Geometry: final body of the model. Coordinates: model frame, mm. Round coordinates to 2 decimals unless told otherwise and drop trailing zeros. Loops run counter-clockwise (first coordinate to the right, second up) from the corner with the lowest first, then second, coordinate; pieces in that order, holes last. Notation, with made-up numbers: (89, 26.5) -> (96, 26.5) arc R12 ccw to (96, 30.5) -> close; hole circle Ø3 at (83.25, 12.25). An arc over 180 degrees is marked (long way). Answer in a Markdown table with one row per item.
```python
from build123d import *

# Parameters (mm, degrees)
F0_W     = 146.750048
F0_H     = 97.573176
F1_DEPTH = 63.5
F3_DEPTH = 97.574176
F5_DEPTH = 97.574176


with BuildPart() as f1:
    # F0 (on Top) → F1 (new body)
    with BuildSketch(Plane.XY):
        Rectangle(F0_W, F0_H)
    extrude(amount=F1_DEPTH)

    # F2 (on face) → F3 (cut, through all)
    with BuildSketch(Plane.XZ.offset(48.786588)):
        Polygon((73.375024, 63.5), (0, 63.5), (73.375024, 0), align=None)
    extrude(amount=-F3_DEPTH, mode=Mode.SUBTRACT)

    # F4 (on face) → F5 (cut, through all)
    with BuildSketch(Plane.XZ.offset(48.786588)):
        Polygon((0, 63.5), (59.064299, 0), (73.375024, 0), align=None)
    extrude(amount=-F5_DEPTH, mode=Mode.SUBTRACT)


solid = f1.part
```
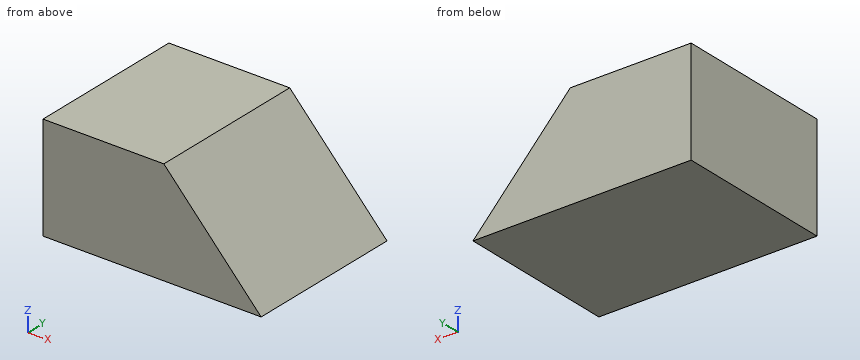
Item 1: Cut plane B-B (x = 51). Output: boundary loops of the cut face in (y, z), then the cut area to 3 significant figures.
Answer:
| item | result |
|---|---|
| outline | (-48.79, 0) -> (48.79, 0) -> (48.79, 8.67) -> (-48.79, 8.67) -> close |
| area | 846 mm² |
Item 2: Line query: probe 1 along X at (y, z) = (2.5, 31); probe 2 along X at (y, z) = (-21, 55); probe 3 along Z at (x, y) = (35.5, 24.5). Output: solid intervals per line, ascending. Write a range as [from, to].
Answer:
| item | result |
|---|---|
| probe 1 | x = [-73.38, 30.23] |
| probe 2 | x = [-73.38, 7.91] |
| probe 3 | z = [0, 25.33] |
Item 3: Cut plane A-A (y = -14). Output: boundary loops of the cut face in (x, z).
Answer:
| item | result |
|---|---|
| outline | (-73.38, 0) -> (59.06, 0) -> (0, 63.5) -> (-73.38, 63.5) -> close |
Item 4: Pin query (flat end, axial travel): pin 1 Ø4 at (x, y) = (6.5, -1) entering from +Z; pin 2 Ø1 at (x, y) = (21, -8) entering from +Z. Return the tip coordinate at first contact, or that it passes through.
Answer:
| item | result |
|---|---|
| pin 1 | stops at z = 58.66 |
| pin 2 | stops at z = 41.46 |
